Geometry: see drawing. Coordinates: mm, zero at the bounding-box minimum. A direction names the side the tool comes from. Coordinates: 2 decimals unless noted, no trailing zeros. Loops run counter-clockwise (first coordinate to the right, second up) from the corner with the lowest first, then second, coordinate; pieces in that order, holes last. Notation, with made-up numbers: (52, 78) - (59, 78) arc R20 cw to (59, 101) - close; hole circle Ø11 at (-29, 66.5). An arc over 180 degrees is marked (long way). Answer in a Markdown table with one row per item.
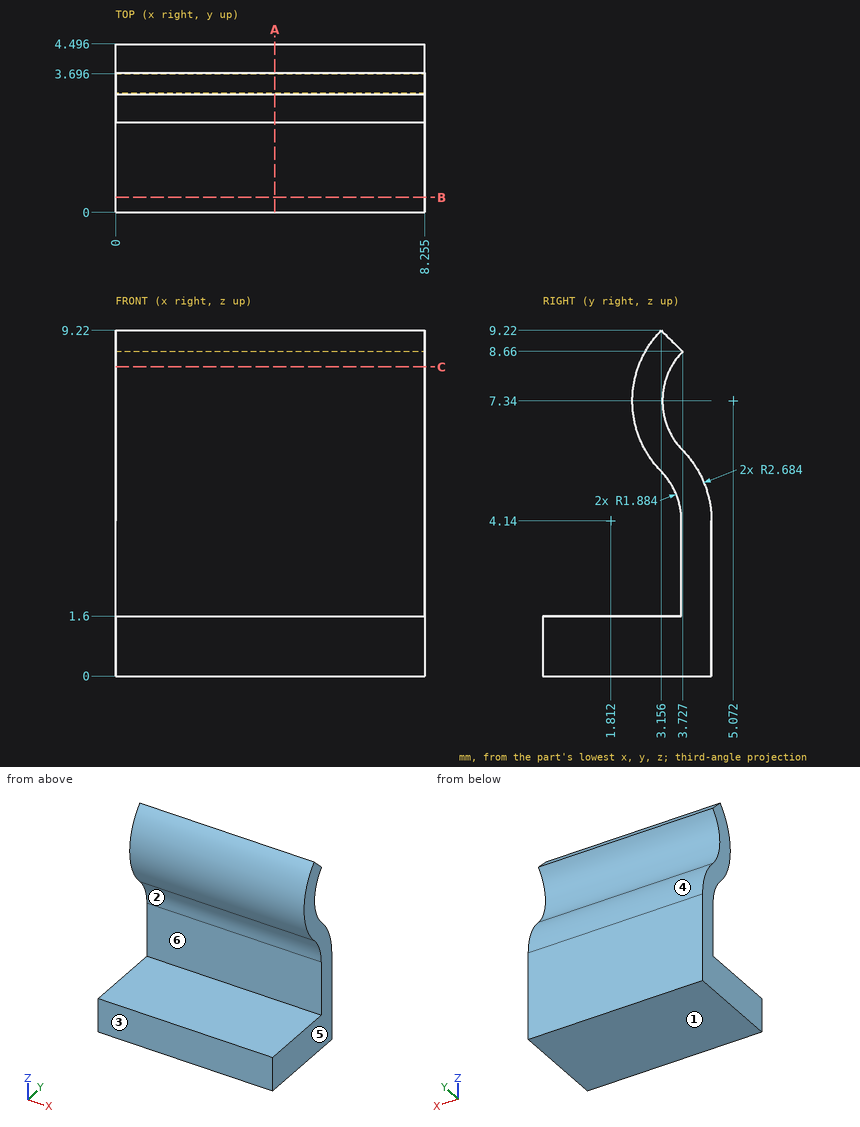
(1) Ray query, probe 1 along Y at (x, z) = (3.5, 3.75) (1 decimal); probe 2 along Z at (x, y) = (6.75, 2); probe 3 along Z at (x, y) = (3.75, 3.95) (1 decimal). Return the intervals inside material, ascending.
Verdict:
| item | result |
|---|---|
| probe 1 | y = 3.7 to 4.5 |
| probe 2 | z = 0 to 1.6 |
| probe 3 | z = 0 to 5.8 |
(2) Cut plane B-B on y = 0.4. Output: boundary loops of the cut face in (x, z) (1 decimal).
Verdict:
| item | result |
|---|---|
| outline | (0, 0) - (8.3, 0) - (8.3, 1.6) - (0, 1.6) - close |
(3) Cut plane A-A on x = 4.25. Output: boundary loops of the cut face in (y, z) (1 decimal).
Verdict:
| item | result |
|---|---|
| outline | (0, 0) - (4.5, 0) - (4.5, 4.1) arc R2.7 ccw to (3.7, 6) arc R1.9 cw to (3.7, 8.7) - (3.2, 9.2) arc R2.7 ccw to (3.2, 5.5) arc R1.9 cw to (3.7, 4.1) - (3.7, 1.6) - (0, 1.6) - close |
(4) Access query for the marked faces 5 and 6. Directions: +Z, -Z, +X, -X, +Y, -Y. A direction counts if a zero-diameter tool reaches every point of the face in a straight line with its end or side. Return the directions, or none.
Verdict:
| item | result |
|---|---|
| face 5 | +Z, -Z, +X, +Y, -Y |
| face 6 | +X, -X, -Y |
(5) First-contact query: pin 1 Ø1.5 at (x, z) = (1, 6) entering from -Y; pin 2 Ø1.8 at (x, y) = (2.5, 2) entering from +Z (1 decimal); pin 3 Ø3 at (x, z) = (6, 2.5) entering from -Y. Flat tips, straight axial feed; report the tip coordinate or a pass-through.
Verdict:
| item | result |
|---|---|
| pin 1 | stops at y = 2.45 |
| pin 2 | stops at z = 8.9 |
| pin 3 | stops at y = 0 |
(6) Pull-direction query (Z, two-part tool) for the marked faces 1, 2, 3 and 4; classes: pulls with the +Z half, pulls with the -Z half, needs draft (parallel to the pull), parting line crosses it, or undercut.
Verdict:
| item | result |
|---|---|
| face 1 | pulls with the -Z half |
| face 2 | undercut |
| face 3 | needs draft |
| face 4 | pulls with the +Z half |
(7) Cut plane C-C on z = 8.25. Output: boundary loops of the cut face in (x, y) (1 decimal).
Verdict:
| item | result |
|---|---|
| outline | (0, 2.5) - (8.3, 2.5) - (8.3, 3.4) - (0, 3.4) - close |
